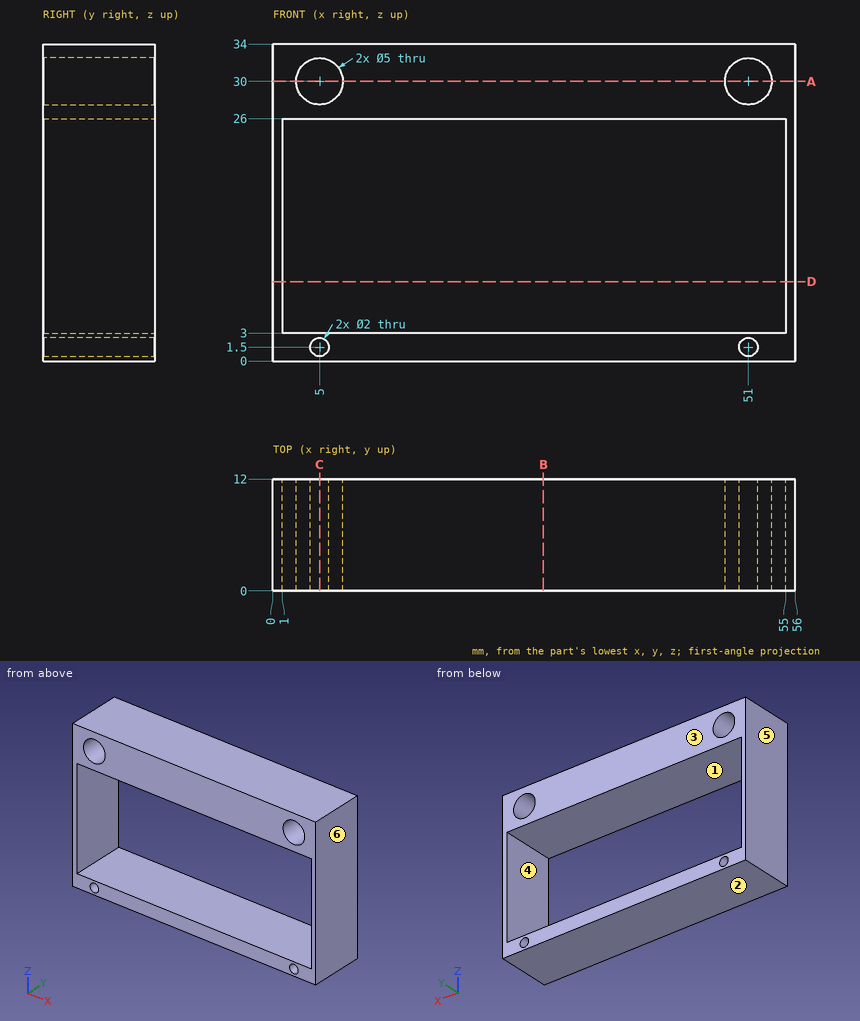
Drawing for the job (mm, zero at the part's lowest x, y, z). A direction names the side the tool comes from. Give positions to 0.01 mm unless a question says otherwise; leave off trailing zeros. Order: outer loops, then holes, each group sorted by start corner. A loop starts at its lowest first (then second) coordinate and runs counter-clockwise, first axis right, second up. Notation, with made-up numbers: M 69.25,-10 L 107.25,-10 A19 ccw 107.25,10 Z; hole C 47.5,6.5 d7. An arc over 180 degrees is marked long. Use a Markdown table: item, result. Add a question column.
(1) Saw through at B-B, the plane x = 29. Give the cut face in (y, z).
(2) Saw through at D-D, the plane z = 8.5. Give the cut face in (x, y), and give its area (3 significant figures).
(3) 3-axis set-ups, long thin cutter, end or side, ignore diameter. For the marked faces 1 and 2: which of +Z, -Z, +X, -X, +Y, -Y reach the whole face in a straight line?
(4) Probe line 1 along X through (y, z) = (8.75, 30); line 2 along Z through (x, y) = (40, 3); line 3 along X through (y, z) = (4, 1.5). List the from-to ranges inside material, lowest first. Write a range as [from, to].
(5) Saw through at C-C, the plane x = 5. Give the cut face in (y, z), and give its area (3 significant figures).
(6) Drop a flat-ended pin along its axis: P1, Ø6, axis at x = 5, z = 30, coming from the +Y side. Give the stop position or say it passes through.
(7) Saw through at A-A, the plane z = 30. Give the cut face in (x, y), and give its area (3 significant figures).
(8) Mould opens along X. For the marked faces 3, 4, 5 and 6 say: +X half, -X half, draft (parallel to the pull), parting line (faces both ways), or undercut.
Answer key:
| question | item | result |
|---|---|---|
| 1 | outline | M 0,0 L 12,0 L 12,3 L 0,3 Z; M 0,26 L 12,26 L 12,34 L 0,34 Z |
| 2 | outline | M 0,0 L 1,0 L 1,12 L 0,12 Z; M 55,0 L 56,0 L 56,12 L 55,12 Z |
| 2 | area | 24.0 mm^2 |
| 3 | face 1 | +Y, -Y |
| 3 | face 2 | -Z, +X, -X, +Y, -Y |
| 4 | line 1 | [0, 2.5], [7.5, 48.5], [53.5, 56] |
| 4 | line 2 | [0, 3], [26, 34] |
| 4 | line 3 | [0, 4], [6, 50], [52, 56] |
| 5 | outline | M 0,0 L 12,0 L 12,0.5 L 0,0.5 Z; M 0,2.5 L 12,2.5 L 12,3 L 0,3 Z; M 0,26 L 12,26 L 12,27.5 L 0,27.5 Z; M 0,32.5 L 12,32.5 L 12,34 L 0,34 Z |
| 5 | area | 48.0 mm^2 |
| 6 | P1 | y = 12 |
| 7 | outline | M 0,0 L 2.5,0 L 2.5,12 L 0,12 Z; M 7.5,0 L 48.5,0 L 48.5,12 L 7.5,12 Z; M 53.5,0 L 56,0 L 56,12 L 53.5,12 Z |
| 7 | area | 552 mm^2 |
| 8 | face 3 | draft |
| 8 | face 4 | undercut |
| 8 | face 5 | -X half |
| 8 | face 6 | +X half |
